Geometry check sheet. Reference: drawing and pictorial views, mm from the part's lowest x, y, z. A direction names the side the tool comes from. Give positions to 0.01 mm unless a question says otherwise; leave off trailing zeros. Order: outer loops, then holes, each group sorted by start corner. A loop starts at its lowest first (then second) coordinate and runs counter-clockwise, first axis right, second up.
Item 1: Sectioned sample at A-A on y = 34.5. Record the boundary of the cut face in (x, z).
Item 2: Sectioned sample at D-D on z = 89.5. Record the boundary of the cut face in (x, y).
Item 3: Sectioned sample at C-C on z = 24.5. Record the boundary of the cut face in (x, y), and give its area (3 significant figures).
Item 4: Material ranges on line 1 along Z through (x, y) = (25, 29); line 2 along Y through (x, z) = (35.5, 8.5); line 3 along Y through (x, z) = (61, 25), recorded low to high.
Item 5: Gauge pin test, flat ends, axial feed: P1, Ø2, axis at x = 58.5, z = 20, coming from the +Y side; P2, Ø3, axis at x = 42.5, z = 35.5, coming from the +Y side; P3, Ø17.5, axis at x = 35, y = 20.5, coming from the +Z side. Record the tip position at first contact, or that the pin passes through.
Item 6: Access from +Z, -Z, +X, -X, +Y, -Y to the whole of each face (thin tool, end or side, straight path). Record for the marked faces 1 and 2.
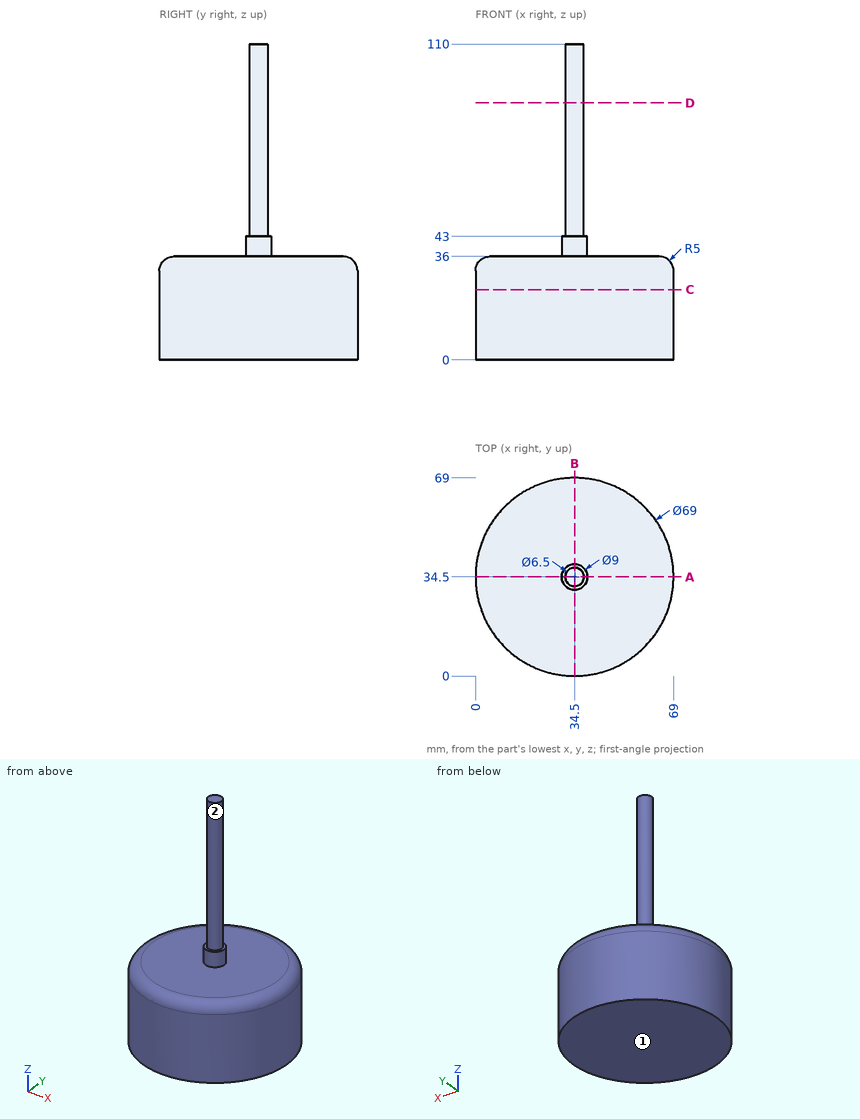
Report:
1. outline: (0, 0) - (69, 0) - (69, 31) arc R5 ccw to (64, 36) - (39, 36) - (39, 43) - (37.75, 43) - (37.75, 110) - (31.25, 110) - (31.25, 43) - (30, 43) - (30, 36) - (5, 36) arc R5 ccw to (0, 31) - close
2. outline: circle Ø6.5 at (34.5, 34.5)
3. outline: circle Ø69 at (34.5, 34.5)
3. area: 3,740 mm2
4. line 1: z = 0 to 36
4. line 2: y = 0.01 to 68.99
4. line 3: y = 12.41 to 56.59
5. P1: stops at y = 60.21
5. P2: stops at y = 67.08
5. P3: stops at z = 36
6. face 1: -Z, +X, -X, +Y, -Y
6. face 2: +Z
